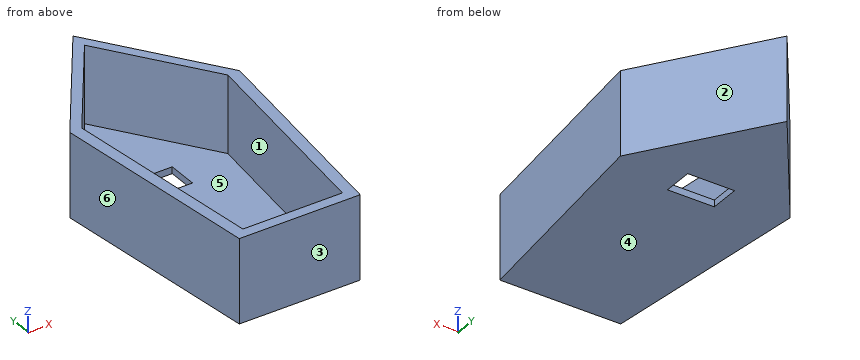
from build123d import *

# Parameters (mm, degrees)
F0_W     = 22.86
F0_H     = 93.98
F1_DEPTH = 31.75
F3_DEPTH = 29.21
F5_DEPTH = 25.4


with BuildPart() as f1:
    # F0 (on Top) → F1 (new body)
    with BuildSketch(Plane.XY):
        Polygon((-25.061955, -44.999161), (-25.061955, 48.980839), (-2.201955, 48.980839), (-2.201955, 82.000839), (-34.44485, 36.017679), align=None)
        with Locations((-13.631955, 1.990839)):
            Rectangle(F0_W, F0_H)
        Polygon((-2.201955, 82.000839), (-2.201955, 48.980839), (20.658045, 48.980839), (20.658045, -44.999161), (29.784556, 36.017679), align=None)
        with Locations((9.228045, 1.990839)):
            Rectangle(F0_W, F0_H)
    extrude(amount=F1_DEPTH)

    # F2 (on face) → F3 (cut)
    with BuildSketch(Plane.XY.offset(31.75)):
        Polygon((25.300306, 36.017679), (-2.201955, 75.554371), (-29.924656, 36.017679), (-21.003638, -41.011075), (16.62305, -41.011075), align=None)
    extrude(amount=-F3_DEPTH, mode=Mode.SUBTRACT)

    # F4 (on face) → F5 (cut)
    with BuildSketch(Plane.XY.offset(2.54)):
        Polygon((6.549126, 39.358769), (-2.201955, 39.358769), (-11.173476, 39.358769), (-11.173476, 27.984561), (6.549126, 27.984561), align=None)
    extrude(amount=-F5_DEPTH, mode=Mode.SUBTRACT)


solid = f1.part
Read the model definition and answer for the solid it produces. Units are mm, in the model's axes. Face numbers are marked on the shaded views. A direction names the side the tool comes from. Round coordinates to 2 decimals unless told otherwise and drop trailing zeros. Loops run counter-clockwise (first coordinate to the right, second up) from the corner with the lowest first, then second, coordinate; pieces in that order, holes last.
Q1. Section B-B on x = 4.5 is taken. Write down the section's boundary in (y, z), and give its area (3 significant figures).
Q2. Section A-A on y = 31.5 is taken. Write down the section's boundary in (x, z).
Q3. Section D-D on y = 49 is taken. Write down the section's boundary in (x, z).
Q4. Which of the six approach directions +Z, -Z, +X, -X, +Y, -Y give full straight-line access (tool end or side, diameter ignored) to the marked faces 5 and 6?
Q5. Consider probe 1 along X at (y, z) = (36, 14.5); probe 2 along Z at (x, y) = (-4, 63); probe 3 along Y at (x, z) = (-1.5, 4.5). Determine where each line is inside the solid, lowest interval first.
Q6. Determine the mould class of the marked faces 1, 2, 3 and 4 for opening direction Y: released by +Y, released by -Y, zero draft, split by the parting line, or undercut.
Q7. Section C-C on z = 13 is taken. Write down the section's boundary in (x, y).
Q8. Each of these flat-tipped pins is pushed along its axis until it touches: pin 1 (1.5 mm diameter, centred on y = -23, z = 5.5, fed in from +X); pin 2 (6 mm diameter, centred on x = -19.5, z = 3.5, fed in from +Y); pin 3 (3 mm diameter, centred on y = 32, z = 1.5, fed in from +X); pin 4 (6 mm diameter, centred on x = -2, y = 7, fed in from -Z). Where does it stop, or does it pass through?
Output:
1. outline: (-45, 0) - (27.98, 0) - (27.98, 2.54) - (-41.01, 2.54) - (-41.01, 31.75) - (-45, 31.75) - close; (39.36, 0) - (72.37, 0) - (72.37, 31.75) - (65.92, 31.75) - (65.92, 2.54) - (39.36, 2.54) - close
1. area: 574 mm2
2. outline: (-33.92, 0) - (-11.17, 0) - (-11.17, 2.54) - (-29.4, 2.54) - (-29.4, 31.75) - (-33.92, 31.75) - close; (6.55, 0) - (29.28, 0) - (29.28, 31.75) - (24.79, 31.75) - (24.79, 2.54) - (6.55, 2.54) - close
3. outline: (-25.34, 0) - (20.75, 0) - (20.75, 31.75) - (16.27, 31.75) - (16.27, 2.54) - (-20.82, 2.54) - (-20.82, 31.75) - (-25.34, 31.75) - close
4. face 5: +Z
4. face 6: +Z, -Z, -X, -Y
5. probe 1: x = -34.44 to -29.92, 25.3 to 29.78
5. probe 2: z = 0 to 2.54
5. probe 3: y = -45 to -41.01, 74.55 to 80.99
6. face 1: undercut
6. face 2: released by +Y
6. face 3: released by -Y
6. face 4: zero draft
7. outline: (-34.44, 36.02) - (-25.06, -45) - (20.66, -45) - (29.78, 36.02) - (-2.2, 82) - close; hole (-29.92, 36.02) - (-21, -41.01) - (16.62, -41.01) - (25.3, 36.02) - (-2.2, 75.55) - close
8. pin 1: stops at x = 23.22
8. pin 2: stops at y = 61.61
8. pin 3: stops at x = 29.5
8. pin 4: stops at z = 0
